Can you work these out from the model? Positions are in its coordinate system, mm. Face numbers are marked on the shaded views. A direction names the side the tool comes from. Coordinates: 2 decimals unless noted, no trailing zeros. Loops run counter-clockwise (first coordinate to the right, second up) from the corner with the lowest first, then second, coordinate; pieces in that order, holes last.
```python
from build123d import *

# Parameters (mm, degrees)
SKETCH_2_W             = 64.02174429
SKETCH_2_H             = 9.248919907
CUT_EXTRUDE_1_DEPTH    = 49
HOLE_WIZARD_M4_2_D     = 3.3
HOLE_WIZARD_M4_2_DEPTH = 5.5
HOLE_WIZARD_M4_2_TIP   = 0.991420021
HOLE_WIZARD_M6_2_D     = 5
HOLE_WIZARD_M6_2_DEPTH = 5.5
HOLE_WIZARD_M6_2_TIP   = 1.502151548


with BuildPart() as part:
    # 草图1 → 旋转1 (revolve)
    with BuildSketch(Plane(origin=(0, 0, 0), x_dir=(1, 0, 0), z_dir=(0, 1, 0)), mode=Mode.PRIVATE) as revolve_1_sk:
        Polygon((20, 7.5), (20, -7.5), (11.1, -7.5), (11.1, -3), (11.7, -3), (11.7, -2), (9.25, -2), (9.25, 2), (11.7, 2), (11.7, 3), (11.1, 3), (11.1, 7.5), align=None)
    revolve(revolve_1_sk.sketch.rotate(Axis((0, 0, -31.9390681), (0, 0, 1)), 180), axis=Axis((0, 0, -31.9390681), (0, 0, 1)))  # turned: the seam where the file's is

    # 草图2 → 切除-拉伸1 (cut)
    with BuildSketch(Plane.XY.offset(7.5)):
        with Locations((-1.141100508, 23.424459954)):
            Rectangle(SKETCH_2_W, SKETCH_2_H)
        with Locations((-1.141100508, -23.424459954)):
            Rectangle(SKETCH_2_W, SKETCH_2_H)
    extrude(amount=-CUT_EXTRUDE_1_DEPTH, mode=Mode.SUBTRACT)

    # M4 螺纹孔2
    with Locations(Plane(origin=(0, 18.8, 0), x_dir=(1, 0, 0), z_dir=(0, 1, 0))):
        with Locations((0, 0)):
            Hole(HOLE_WIZARD_M4_2_D / 2, depth=HOLE_WIZARD_M4_2_DEPTH)
            with Locations((0, 0, -(HOLE_WIZARD_M4_2_DEPTH + HOLE_WIZARD_M4_2_TIP / 2))):  # 118° drill point
                Cone(0, HOLE_WIZARD_M4_2_D / 2, HOLE_WIZARD_M4_2_TIP, mode=Mode.SUBTRACT)

    # M6 螺纹孔2
    with Locations(Plane(origin=(0, -18.8, 0), x_dir=(-1, 0, 0), z_dir=(0, -1, 0))):
        with Locations((0, 0)):
            Hole(HOLE_WIZARD_M6_2_D / 2, depth=HOLE_WIZARD_M6_2_DEPTH)
            with Locations((0, 0, -(HOLE_WIZARD_M6_2_DEPTH + HOLE_WIZARD_M6_2_TIP / 2))):  # 118° drill point
                Cone(0, HOLE_WIZARD_M6_2_D / 2, HOLE_WIZARD_M6_2_TIP, mode=Mode.SUBTRACT)


solid = part.part
```
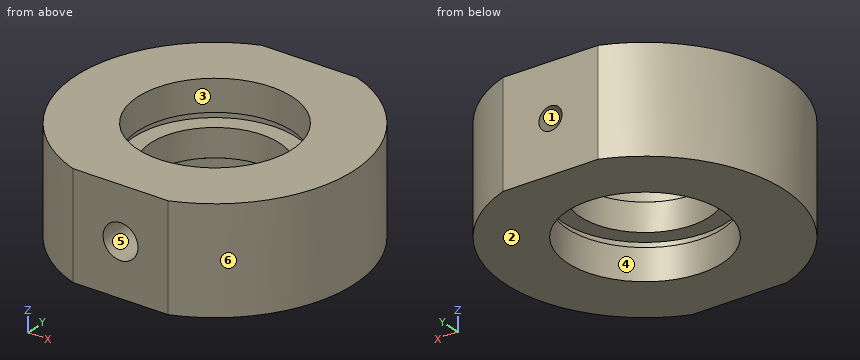
(1) If we mould it in two halves opening along Z, with no side actions, what happens to the marked faces 1, 2 and 3? For each: released by +Z, released by -Z, zero draft, split by the parting line, or undercut.
Check values:
face 1: undercut
face 2: released by -Z
face 3: zero draft
(2) I want a section at C-C on x = 4. Write out the boundary of the cut face in (y, z) (3 decimals), then the cut area to 3 significant figures.
Check values:
outline: (-18.8, -7.5) - (-10.354, -7.5) - (-10.354, -3) - (-10.995, -3) - (-10.995, -2) - (-8.34, -2) - (-8.34, 2) - (-10.995, 2) - (-10.995, 3) - (-10.354, 3) - (-10.354, 7.5) - (-18.8, 7.5) - close; (8.34, -2) - (10.995, -2) - (10.995, -3) - (10.354, -3) - (10.354, -7.5) - (18.8, -7.5) - (18.8, 7.5) - (10.354, 7.5) - (10.354, 3) - (10.995, 3) - (10.995, 2) - (8.34, 2) - close
area: 267 mm2
(3) I want a section at B-B on z = -5.75. Write out the boundary of the cut face in (x, y), then the cut area to 3 significant figures.
Check values:
outline: (-6.82, -18.8) - (6.82, -18.8) arc R20 ccw to (6.82, 18.8) - (-6.82, 18.8) arc R20 ccw to start; hole circle Ø22.2 at (0, 0)
area: 848 mm2
(4) I want a section at A-A on y = 0. Write out the boundary of the cut face in (x, z), then the cut area to 3 significant figures.
Check values:
outline: (-20, -7.5) - (-11.1, -7.5) - (-11.1, -3) - (-11.7, -3) - (-11.7, -2) - (-9.25, -2) - (-9.25, 2) - (-11.7, 2) - (-11.7, 3) - (-11.1, 3) - (-11.1, 7.5) - (-20, 7.5) - close; (9.25, -2) - (11.7, -2) - (11.7, -3) - (11.1, -3) - (11.1, -7.5) - (20, -7.5) - (20, 7.5) - (11.1, 7.5) - (11.1, 3) - (11.7, 3) - (11.7, 2) - (9.25, 2) - close
area: 279 mm2
(5) If I drill on probe 1 along Y at (x, z) = (0, 6.4); probe 2 along Z at (x, y) = (0, 15); probe 3 along Y at (x, z) = (0, 2.7), over which ranges is the centre line in solid material (lowest first)?
Check values:
probe 1: y = -18.8 to -11.1, 11.1 to 18.8
probe 2: z = -7.5 to -1.65, 1.65 to 7.5
probe 3: y = -18.8 to -11.7, 11.7 to 18.8
(6) I'm going to push flat-ended pins straight in: pin 1 (11.5 mm diameter, centred on x = -2, y = 1.5, fed in from -Z); pin 2 (3 mm diameter, centred on y = 5, z = 1, fed in from -X); pin 3 (1.5 mm diameter, centred on y = 9, z = 3, fed in from -X); pin 4 (8 mm diameter, centred on x = 13, z = 3, fed in from +Y). Where does each tip first touch, or does it pass through?
Check values:
pin 1: passes through
pin 2: stops at x = -19.69
pin 3: stops at x = -18.22
pin 4: stops at y = 17.86
(7) Which directions (+Z, -Z, +X, -X, +Y, -Y) give clear straight access to the entire face, cutting with the end or side of a thin tool? Please do the marked faces 4, 5 and 6.
Check values:
face 4: -Z
face 5: -Y
face 6: +Z, -Z, +X
(8) I want a section at D-D on y = -15. Write out the boundary of the cut face in (x, z), then the cut area to 3 significant figures.
Check values:
outline: (-13.23, -7.5) - (13.23, -7.5) - (13.23, 7.5) - (-13.23, 7.5) - close; hole circle Ø5 at (0, 0)
area: 377 mm2
